Job drawing, mm, ordinate dimensions from the low corner. One solid piece. A direction names the side the tool comes from. Coordinates: 2 decimals unless noted, no trailing zeros. Write each loop counter-clockwise with the first axis right and the second up, starting at its lowest first coordinate (ties: lowest second). Pieces come first, ordered by that corner, then holes.
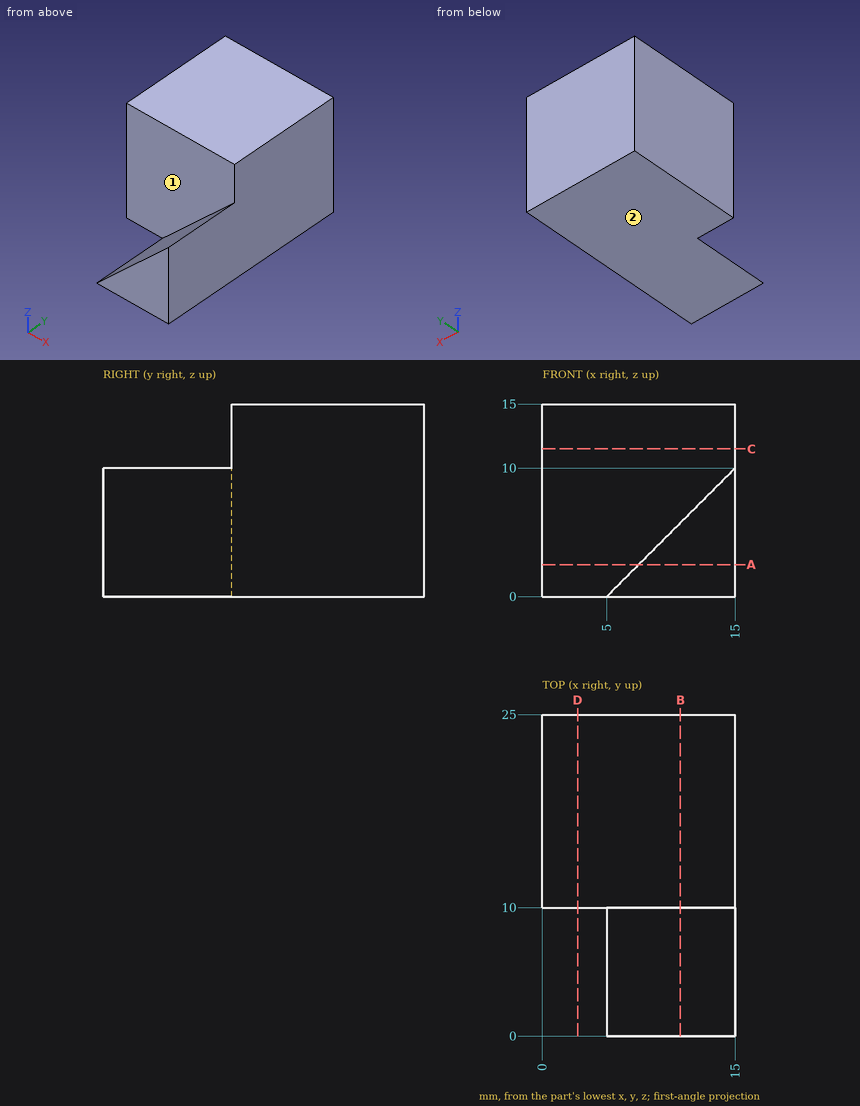
1. Probe line 1 along Y through (x, z) = (5, 3.5); line 2 along X through (y, z) = (5, 8.25); line 3 along Z through (x, y) = (11.75, 8.5). List the from-to ranges inside material, lowest first.
Computed values:
line 1: y = 10 to 25
line 2: x = 13.25 to 15
line 3: z = 0 to 6.75
2. Saw through at A-A on z = 2.5. List the corners of the cut face in (x, y).
Computed values:
outline: (0, 10) - (7.5, 10) - (7.5, 0) - (15, 0) - (15, 25) - (0, 25) - close
3. 3-axis set-ups, long thin cutter, end or side, ignore diameter. For the marked faces 1 and 2: which of +Z, -Z, +X, -X, +Y, -Y reach the whole face in a straight line?
Computed values:
face 1: +Z, -X, -Y
face 2: -Z, +X, -X, +Y, -Y
4. Saw through at B-B on x = 10.75. List the corners of the cut face in (y, z), plus the area to 4 significant figures.
Computed values:
outline: (0, 0) - (25, 0) - (25, 15) - (10, 15) - (10, 5.75) - (0, 5.75) - close
area: 282.5 mm2
5. Saw through at C-C on z = 11.5. List the corners of the cut face in (x, y), plus the area to 3 significant figures.
Computed values:
outline: (0, 10) - (15, 10) - (15, 25) - (0, 25) - close
area: 225 mm2
6. Flat gauge pins, fed straight in: pin 1 (3 mm diameter, centred on y = 20.5, z = 13, fed in from -X); pin 2 (4.5 mm diameter, centred on x = 4.5, z = 5, fed in from -Y). Where does each tip first touch, or does it go through?
Computed values:
pin 1: stops at x = 0
pin 2: stops at y = 10
7. Saw through at D-D on x = 2.75. List the corners of the cut face in (y, z).
Computed values:
outline: (10, 0) - (25, 0) - (25, 15) - (10, 15) - close
